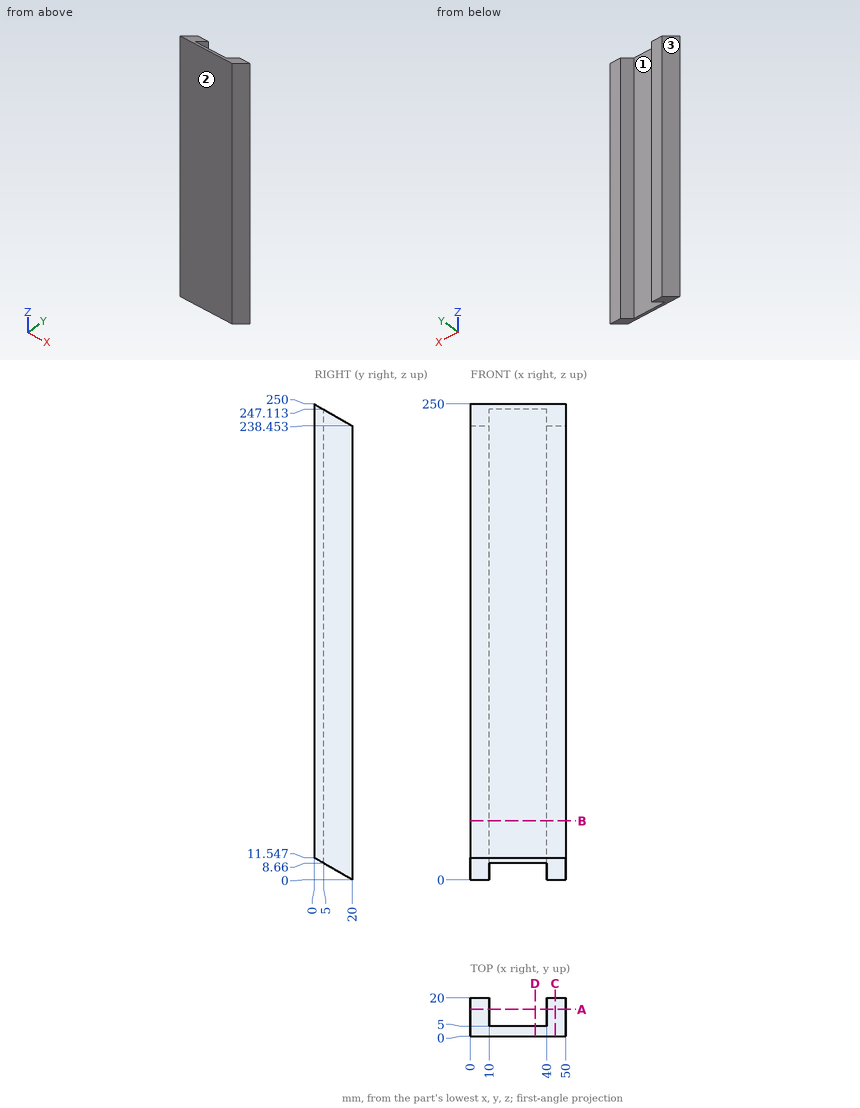
For this review, use the dimensioned drawing (mm, ordinates from the lowest corner) and the shaded views. Coordinates: 2 decimals unless noted, no trailing zeros. Loops run counter-clockwise (first coordinate to the right, second up) from the corner with the lowest first, then second, coordinate; pieces in that order, holes last. Notation, with made-up numbers: (78, -13.75) -> (85, -13.75) arc R18 ccw to (85, -2.75) -> close; hole circle Ø11 at (-8.5, 77). An arc over 180 degrees is marked (long way). Use a Markdown table: item, result. Add a question column.
1. To check wall thickness, follow line 1 (X direction, y = 10.75, z = 114.5); line 2 (Y direction, x = 38, z = 167); line 3 (Z direction, x = 13, y = 2.5). State the ranges of each line that lie inside material, in increasing order.
2. Add section B-B on z = 31. Write out the cut boundary in (x, y).
3. Add section A-A on y = 14. Write out the cut boundary in (x, z).
4. Add section D-D on x = 34. Write out the cut boundary in (y, z).
5. Draft analysis for pull direction X (two halves, no side actions). For the marked faces 1, 2 and 3, state which applies: pulls with the +X half, pulls with the -X half, needs draft (parallel to the pull), parting line crosses it, or undercut.
6. Add section C-C on x = 44.5. Write out the cut boundary in (y, z).
7. Clearance check with a flat-ended pin moving along its axis: pin 1 Ø24 at (x, z) = (24, 180.5) entering from +Y. State where the tip first meets the part, or that it passes through.
Returned:
| question | item | result |
|---|---|---|
| 1 | line 1 | x = 0 to 10, 40 to 50 |
| 1 | line 2 | y = 0 to 5 |
| 1 | line 3 | z = 10.1 to 248.56 |
| 2 | outline | (0, 0) -> (50, 0) -> (50, 20) -> (40, 20) -> (40, 5) -> (10, 5) -> (10, 20) -> (0, 20) -> close |
| 3 | outline | (0, 3.46) -> (10, 3.46) -> (10, 241.92) -> (0, 241.92) -> close; (40, 3.46) -> (50, 3.46) -> (50, 241.92) -> (40, 241.92) -> close |
| 4 | outline | (0, 11.55) -> (5, 8.66) -> (5, 247.11) -> (0, 250) -> close |
| 5 | face 1 | undercut |
| 5 | face 2 | needs draft |
| 5 | face 3 | pulls with the -X half |
| 6 | outline | (0, 11.55) -> (20, 0) -> (20, 238.45) -> (0, 250) -> close |
| 7 | pin 1 | stops at y = 5 |
